For this review, take the finished solid that the model builds, in its own axes (mm). Coordinates: 2 decimals unless noted, no trailing zeros. Loops run counter-clockwise (first coordinate to the right, second up) from the corner with the lowest first, then second, coordinate; pieces in that order, holes last. Notation, with made-up numbers: M 55,16.5 L 102,16.5 A24 cw 102,28.5 Z; hole C -23,73.25 d6. An arc over 180 degrees is marked long. Use one line per item in the form item = value.
Solid Edge part; units mm, degrees
sketch "Sketch1" plane through (0, 0, 0) normal (0, -1, 0) x (1, 0, 0)
  line L0 (-27.5, -7.5) -> (27.5, -7.5)
  line L1 (27.5, -7.5) -> (27.5, 7.5)
  line L2 (27.5, 7.5) -> (-27.5, 7.5)
  line L3 (-27.5, 7.5) -> (-27.5, -7.5)
  dimension "D1" = 27.5
  dimension "D2" = 27.5
extrude "ExtrudedProtrusion_1" add sketch "Sketch1" along normal blind 3 and the other way blind 3
fillet "Round_1" radius 7.5 4 edges at (27.5, 0, 7.5) (27.5, 0, -7.5) (-27.5, 0, 7.5) (-27.5, 0, -7.5)
hole "Hole_1" at (21.9203, -3, 0) direction (0, 1, 0) diameter 3.6 end up to next start chamfer 0.3 start chamfer angle 30 end chamfer 0.3 end chamfer angle 30
hole "Hole1" at (-21.9203, -3, 0) direction (0, 1, 0) diameter 3.6 end up to next start chamfer 0.3 start chamfer angle 30 end chamfer 0.3 end chamfer angle 30
fillet "Round_2" radius 1 7 edges at (0, -3, -7.5) (27.5, -3, 0) (0, -3, 7.5) (-27.5, -3, 0) (-27.5, 3, 0) (0, 3, 7.5) (0, 3, -7.5)
hole "Hole_3" at (0, -3, 0) direction (0, 1, 0) diameter 9 end up to next start chamfer 0.6 start chamfer angle 30 end chamfer 0.6 end chamfer angle 30
properties material "Polyethylene, low density"
1. Consider section B-B on y = 1. State how many separate pieces and enclosed holes the cut face has, plus the area to 3 significant figures.
Computed values:
separate_pieces = 1
enclosed_holes = 3
area = 693 mm2
2. For pin 1 Ø3 at (y, z) = (0, -2.5) entering from -X; pin 2 Ø3 at (x, z) = (-21.92, 0) entering from +Y; pin 3 Ø3 at (y, z) = (-1, 4) entering from +X, all flat-tipped, find the tip position at first contact; note any pin that passes through.
Computed values:
pin_1 = -27.43
pin_2 = through
pin_3 = 27.07
3. Wall thickness on line 1 along Z through (x, y) = (0, 1); line 2 along Z through (x, y) = (-1, -1); line 3 along X through (y, z) = (-2.25, 5): over which ranges is each line inside the solid? List them lowest first. Write a range as from..to.
Computed values:
line_1 = -7.5..-4.5, 4.5..7.5
line_2 = -7.5..-4.39, 4.39..7.5
line_3 = -25.55..25.55
4. Draft analysis for pull direction X (two halves, no side actions). For faces 1 (the face through (25.362, -0.028, 5.245)), 2 (the face through (23.705, -0.035, 0.234)), 3 (the face through (-0.28, -2.715, 7.199)), state which applies: +X half, -X half, draft (parallel to the pull), parting line (faces both ways), or undercut.
Computed values:
face_1 = +X half
face_2 = undercut
face_3 = draft
5. Consider section A-A on x = 0. Write out the cut boundary in (y, z), plus the area to 3 significant figures.
Computed values:
outline = M -3,-6.5 A1 ccw -2,-7.5 L 2,-7.5 A1 ccw 3,-6.5 L 3,-5.1 L 1.96,-4.5 L -1.96,-4.5 L -3,-5.1 Z; M -3,5.1 L -1.96,4.5 L 1.96,4.5 L 3,5.1 L 3,6.5 A1 ccw 2,7.5 L -2,7.5 A1 ccw -3,6.5 Z
area = 33.9 mm2
